Could you check a few things on this model? Use its own coordinates, in mm. Give positions to 0.01 mm unless a question says otherwise; leave off trailing zeros. Loops run counter-clockwise (first coordinate to the right, second up) from the corner with the lowest first, then second, coordinate; pieces in that order, holes last. Notation, with made-up numbers: M -23,49.25 L -3,49.25 A29 cw -3,81.25 Z; hole C 32.5,76 d8. An arc over 180 degrees is marked long. Answer in a Markdown table with one row per item. Add a question column.
1. I'm going to push flat-ended pins straight in: pin 1 Ø5 at (x, z) = (-11, 15.5) entering from -Y; pin 2 Ø10 at (x, y) = (-9.5, 50) entering from -Z; pin 3 Ø12 at (y, z) = (-13.5, 4.5) entering from -X (3 decimals); pin 4 Ø2.5 at (x, z) = (-23, 8.5) entering from -Y. Where does each tip first touch, or does it pass through?
2. If we section it at C-C on y = 8: List the corners of the cut face in (x, z) for me (3 decimals).
3. Thinking about a two-plate mould opening in X: for faces 1 (the cylindrical face through (-0.489, 57.514, 12.522)), 2 (the flat face through (25.4, -2, 13)), 3 (the flat face through (22.225, -2, 13)), 4 (the flat face through (-24, 35.294, 13)), which applies, released by +X, released by -X, zero draft, split by the parting line, or undercut?
4. I need wall thicknesses on line 1 along X through (y, z) = (-29, 4.5) (3 decimals); line 2 along X through (y, z) = (38.5, 2.75); line 3 along X through (y, z) = (51.5, 5.75). Which ranges of each line are inside material? Lowest first, please. Write a range as from..to.
5. If we section it at A-A on z = 17: List the corners of the cut face in (x, y) for me (3 decimals), then the cut area to 3 significant figures.
6. If we section it at B-B on x = 0: List the corners of the cut face in (y, z) for me.
Autodesk Inventor part; units mm, degrees
ref_plane "YZ Plane" through (0, 0, 0) normal (1, 0, 0) x (0, 1, 0)
ref_plane "XZ Plane" through (0, 0, 0) normal (0, 1, 0) x (-1, 0, 0)
ref_plane "XY Plane" through (0, 0, 0) normal (0, 0, 1) x (1, 0, 0)
sketch "Sketch1" plane through (0, 0, 0) normal (0, 0, 1) x (1, 0, 0)
  arc A0 (25.4, 35.2941) -> (-25.4, 35.2941) centre (0, 35.2941) ccw
  line L0 (25.4, 35.2941) -> (25.4, -40.9059)
  arc A1 (22.225, 35.2941) -> (-22.225, 35.2941) centre (0, 35.2941) ccw
  line L1 (22.225, 35.2941) -> (22.225, -40.9059)
  line L2 (22.225, -40.9059) -> (25.4, -40.9059)
  line L3 (22.225, 35.2941) -> (-22.225, 35.2941) construction
  line L4 (-25.4, 35.2941) -> (-22.225, 35.2941)
  point P0 (0, 0)
  dimension "d0" = 50.8
  dimension "d2" = 76.2
  dimension "d3" = 44.45
extrude "Extrusion1" add sketch "Sketch1" along normal blind 25.4
properties part number "Hook 2.0" material "Aluminum 6061"
Results:
| question | item | result |
|---|---|---|
| 1 | pin 1 | y = 52.95 |
| 1 | pin 2 | z = 0 |
| 1 | pin 3 | x = 22.225 |
| 1 | pin 4 | y = 35.29 |
| 2 | outline | M 22.225,0 L 25.4,0 L 25.4,25.4 L 22.225,25.4 Z |
| 3 | face 1 | undercut |
| 3 | face 2 | released by +X |
| 3 | face 3 | released by -X |
| 3 | face 4 | zero draft |
| 4 | line 1 | 22.225..25.4 |
| 4 | line 2 | -25.2..-21.99, 21.99..25.2 |
| 4 | line 3 | -19.56..-15.21, 15.21..19.56 |
| 5 | outline | M -25.4,35.294 L -22.225,35.294 A22.225 cw 22.225,35.294 L 22.225,-40.906 L 25.4,-40.906 L 25.4,35.294 A25.4 ccw Z |
| 5 | area | 479 mm2 |
| 6 | outline | M 57.52,0 L 60.69,0 L 60.69,25.4 L 57.52,25.4 Z |
